Verification items for the finished model (mm, model axes). A direction names the side the tool comes from. Coordinates: 2 decimals unless noted, no trailing zeros. Order: outer loops, then holes, each group sorted by start corner. A loop starts at its lowest first (then second) coordinate and runs counter-clockwise, first axis right, second up.
Q1. Depth check by flat-ended pin: P1, Ø4, axis at x = 11, y = 6, coming from the -Z side; P2, Ø12, axis at y = -12, z = 85, coming from the +X side; P3, Ø1, axis at x = 11, z = 17, coming from the -Y side; P4, Ø10, axis at x = 15, y = 6, coming from the +Z side. Enter the tip coordinate at first touch or a pass-through.
Q2. Cross-section at C-C, the plane z = 112. Record the boundary of the cut face in (x, y).
Q3. Thickness scan on line 1 (X direction, y = -1, z = 40); line 2 (Y direction, x = 0, z = 89); line 3 (X direction, y = -16.5, z = 5). Record the ranges inside material, lowest first.
Q4. Set-up check for faces 1 (the cylindrical face through (20.03, 6.31, 70.7)), 2 (the flat face through (0, 0, 10)): record each of +Z, -Z, +X, -X, +Y, -Y from which the full face is reachable in a straight line by a thin tool's end or side.
Q5. Cross-section at A-A, the plane y = 0. Record the boundary of the cut face in (x, z), and give its area (3 significant figures).
Q6. Draft check along Y on faces 3 (the flat face through (-5.7, 20.5, 120)), 4 (the cylindrical face through (20.03, -6.31, 3.45)), 5 (the cylindrical face through (23.846, 7.509, 60.681)). Enter one of: pulls with the +Y half, pulls with the -Y half, needs draft (parallel to the pull), parting line crosses it, or undercut.
from build123d import *

# Parameters (mm, degrees)
F0_R     = 25
F1_DEPTH = 120
F2_R     = 21
F3_DEPTH = 100
F4_R     = 21
F5_DEPTH = 10
F6_R     = 3


with BuildPart() as f1:
    # F0 (on Top) → F1 (new body)
    with BuildSketch(Plane.XY):
        Circle(F0_R)
    extrude(amount=F1_DEPTH)

    # F2 (on face) → F3 (cut)
    with BuildSketch(Plane.XY.offset(120)):
        Circle(F2_R)
    extrude(amount=-F3_DEPTH, mode=Mode.SUBTRACT)

    # F4 (on face) → F5 (cut)
    with BuildSketch(Plane(origin=(0, 0, 0), x_dir=(1, 0, 0), z_dir=(0, 0, -1))):
        Circle(F4_R)
    extrude(amount=-F5_DEPTH, mode=Mode.SUBTRACT)

    # F6
    f6_edges = [f1.edges().sort_by_distance(p)[0] for p in [
        (-25, 0, 0),
        (-21, 0, 10),
    ]]
    fillet(f6_edges, radius=F6_R)


solid = f1.part
Check values:
1. P1: stops at z = 10
1. P2: stops at x = 24.27
1. P3: stops at y = -22.69
1. P4: stops at z = 120
2. outline: circle Ø50 at (0, 0); hole circle Ø42 at (0, 0)
3. line 1: x = -24.98 to -20.98, 20.98 to 24.98
3. line 2: y = -25 to -21, 21 to 25
3. line 3: x = -18.78 to -12.99, 12.99 to 18.78
4. face 1: +Z
4. face 2: -Z
5. outline: (-25, 3) arc R3 ccw to (-22, 0) - (-21, 0) - (-21, 7) arc R3 cw to (-18, 10) - (18, 10) arc R3 cw to (21, 7) - (21, 0) - (22, 0) arc R3 ccw to (25, 3) - (25, 120) - (21, 120) - (21, 20) - (-21, 20) - (-21, 120) - (-25, 120) - close
5. area: 1,380 mm2
6. face 3: needs draft
6. face 4: undercut
6. face 5: parting line crosses it
